Here's how the part is built. I have some questions about the finished solid (model axes, mm). Round coordinates to 2 decimals unless told otherwise and drop trailing zeros. Loops run counter-clockwise (first coordinate to the right, second up) from the corner with the lowest first, then second, coordinate; pieces in that order, holes last. Notation, with made-up numbers: M -14,63.25 L -5,63.25 A18 cw -5,72.25 Z; hole C -7,15.25 d6. An arc over 180 degrees is marked long. Use a Markdown table: item, result.
Autodesk Inventor part; units mm, degrees
ref_plane "Arbeitsebene1" through (-7.5, 0, 0) normal (1, 0, 0) x (0, 1, 0)
ref_plane "Arbeitsebene2" through (7.5, 0, 0) normal (1, 0, 0) x (0, 1, 0)
ref_plane "XZ Plane" through (0, 0, 0) normal (0, 1, 0) x (-1, 0, 0)
sketch "Skizze1" plane through (0, 0, 0) normal (0, 1, 0) x (-1, 0, 0)
  circle A0 centre (0, 0) radius 17.5
  dimension "d0" = 35
extrude "Extrusion1" add sketch "Skizze1" along normal blind 724.33
ref_plane "Arbeitsebene1" through (-7.5, 0, 0) normal (1, 0, 0) x (0, 1, 0)
sketch "Skizze2" plane through (-7.5, 0, 0) normal (1, 0, 0) x (0, 1, 0)
  line L0 (0, 0) -> (0, 3.311)
  line L1 (0, -17.5) -> (0, 17.5) construction
  line L2 (0, 0) -> (0, -3.311)
  line L3 (0, 3.311) -> (20, 3.311)
  line L4 (20, 3.311) -> (20, -3.311)
  line L5 (20, -3.311) -> (0, -3.311)
  line L6 (0, -3.311) -> (0, 3.311)
  dimension "d4" = 3.311
  dimension "d5" = 3.311
  dimension "d6" = 20
extrude "Extrusion2" cut sketch "Skizze2" against normal blind 724.33
ref_plane "Arbeitsebene2" through (7.5, 0, 0) normal (1, 0, 0) x (0, 1, 0)
sketch "Skizze3" plane through (7.5, 0, 0) normal (1, 0, 0) x (0, 1, 0)
  line L0 (724.33, -17.5) -> (724.33, 17.5) construction
  line L1 (724.33, 0) -> (724.33, 3.311)
  line L2 (724.33, 0) -> (724.33, -3.311)
  line L3 (724.33, 3.311) -> (704.33, 3.311)
  line L4 (704.33, 3.311) -> (704.33, -3.311)
  line L5 (704.33, -3.311) -> (724.33, -3.311)
  line L6 (724.33, -3.311) -> (724.33, 3.311)
  point P0 (0, 0)
  dimension "d10" = 3.311
  dimension "d11" = 3.311
  dimension "d12" = 20
extrude "Extrusion3" cut sketch "Skizze3" along normal blind 724.33
equation "\"d0\" = Wellensdurchmesser"
equation "\"d7\" = Wellenlänge"
equation "\"d13\" = Wellenlänge"
equation "\"Wellensdurchmesser\" = 35"
equation "\"Wellenlänge\" = 724.33"
properties part number "Welle"
Q1. I need wall thicknesses on line 1 (X direction, y = 309, z = 0.5); line 2 (X direction, y = 585, z = -2.5); line 3 (Z direction, x = 1.5, y = 456). Which ranges of each line are inside material? Lowest first, please. Write a range as from..to.
Return value:
| item | result |
|---|---|
| line 1 | x = -17.49..17.49 |
| line 2 | x = -17.32..17.32 |
| line 3 | z = -17.44..17.44 |
Q2. Imagine slicing it at A-A, the plane y = 530.5. Please give me the cut outline in (x, z).
Return value:
| item | result |
|---|---|
| outline | C 0,0 d35 |
Q3. Will these pins go through, and if not, where does the flat tip stop? P1, Ø7.5, axis at x = 11.5, y = 710, coming from the -Z side; P2, Ø3, axis at x = -12, y = 8, coming from the -Z side; P3, Ø3, axis at x = -14, y = 13, coming from the +Z side.
Return value:
| item | result |
|---|---|
| P1 | stops at z = -15.69 |
| P2 | stops at z = -14 |
| P3 | stops at z = 12.25 |
